```python
from build123d import *

# Parameters (mm, degrees)
F0_W      = 5
F0_H      = 17
F0_H_2    = 8
F0_W_2    = 21
F0_W_3    = 100
F1_DEPTH  = 25
F3_DEPTH  = 8
F4_R      = 2.5
F5_R      = 2.49999
F6_R      = 2.6
F7_DEPTH  = 25
F8_R      = 5
F9_R      = 4.5
F9_R_2    = 2.6
F10_DEPTH = 6
F2_W      = 10
F2_H      = 25
F11_DEPTH = 25
F12_R     = 2


# Not quite as in the source:
# - a fillet or chamfer is up to 0.001 mm smaller than in the source, because OpenCascade refuses the exact size


with BuildPart() as f1:
    # F0 (on Front) → F1 (new body)
    with BuildSketch(Plane.XZ):
        with Locations((-16.2189533483, 16.5)):
            Rectangle(F0_W, F0_H)
        with Locations((-16.2189533483, 4)):
            Rectangle(F0_W, F0_H_2)
        with Locations((-3.2189533483, 4)):
            Rectangle(F0_W_2, F0_H_2)
        with Locations((9.7810466517, 4)):
            Rectangle(F0_W, F0_H_2)
        with Locations((9.7810466517, 16.5)):
            Rectangle(F0_W, F0_H)
        with Locations((62.2810466517, 4)):
            Rectangle(F0_W_3, F0_H_2)
    extrude(amount=F1_DEPTH)

    # F2 (on face) → F3 (join)
    with BuildSketch(Plane.XY.offset(8)):
        Polygon((87.2810466517, -125), (112.2810466517, -125), (112.2810466517, -25), (104.7810466517, -25), (104.7810466517, -115), (94.7810466517, -115), (94.7810466517, -25), (87.2810466517, -25), align=None)
        Polygon((104.7810466517, 0), (112.2810466517, 0), (112.2810466517, 30), (87.2810466517, 30), (87.2810466517, 0), (94.7810466517, 0), (94.7810466517, 20), (104.7810466517, 20), align=None)
    extrude(amount=-F3_DEPTH)

    # F4
    f4_edges = [f1.edges().sort_by_distance(p)[0] for p in [
        (112.281047, -47.5, 0),
        (112.281047, -47.5, 8),
    ]]
    fillet(f4_edges, radius=F4_R)

    # F5 (radius 2.5 in the source; OpenCascade refuses exactly that, so slightly less here)
    f5_edges = [f1.edges().sort_by_distance(p)[0] for p in [
        (12.281047, -12.5, 25),
        (7.281047, -12.5, 25),
        (-18.718953, -12.5, 25),
        (-13.718953, -12.5, 25),
    ]]
    fillet(f5_edges, radius=F5_R)

    # F6 (on face) → F7 (cut)
    with BuildSketch(Plane.XY.offset(8)):
        with Locations((-3.2189533483, -12.5)):
            Circle(F6_R)
    extrude(amount=-F7_DEPTH, mode=Mode.SUBTRACT)

    # F8
    f8_edges = [f1.edges().sort_by_distance(p)[0] for p in [
        (87.281047, 30, 4),
        (87.281047, -125, 4),
    ]]
    fillet(f8_edges, radius=F8_R)

    # F9 (on face) → F10 (cut)
    with BuildSketch(Plane(origin=(0, 0, 0), x_dir=(1, 0, 0), z_dir=(0, 0, -1))):
        with Locations((-3.2189533483, 12.5)):
            Circle(F9_R)
        with Locations((-3.2189533483, 12.5)):
            Circle(F9_R_2, mode=Mode.SUBTRACT)
    extrude(amount=-F10_DEPTH, mode=Mode.SUBTRACT)

    # F2 (on face) → F11 (cut)
    with BuildSketch(Plane.XY.offset(8)):
        with Locations((99.7810466517, -12.5)):
            Rectangle(F2_W, F2_H)
    extrude(amount=-F11_DEPTH, mode=Mode.SUBTRACT)

    # F12
    f12_edges = [f1.edges().sort_by_distance(p)[0] for p in [
        (94.781047, -47.5, 8),
        (99.781047, 20, 8),
        (104.781047, -47.5, 8),
        (99.781047, -115, 8),
        (99.781047, 20, 0),
        (94.781047, -47.5, 0),
        (104.781047, -47.5, 0),
        (99.781047, -115, 0),
    ]]
    fillet(f12_edges, radius=F12_R)


solid = f1.part
```
Model file for the job. Use its own axes, mm. A direction names the side the tool comes from. Coordinates: 2 decimals unless noted, no trailing zeros. Write each loop counter-clockwise with the first axis right and the second up, starting at its lowest first coordinate (ties: lowest second). Pieces come first, ordered by that corner, then holes. Notation, with made-up numbers: (37.5, -20) - (51.5, -20) arc R10 cw to (51.5, -2) - close; hole circle Ø5 at (28.25, -26.75). An arc over 180 degrees is marked (long way). One line per item, written item: value. Start each with the question number.
1. Slice it at D-D (x = 77). Write the cut outline in (y, z), plus the area to 3 significant figures.
2. Tool access for faces 4 (the flat face through (-3.3, -9.6, 6)), 5 (the flat face through (12.281, -12, 15)), 6 (the flat face through (7.281, -12, 15)), 7 (the flat face through (87.281, 13, 4)), 8 (the flat face through (34, -25, 7)): list every direction of +Z, -Z, +X, -X, +Y, -Y with a clear straight run to the whole face (end or side of a thin tool).
3. Slice it at B-B (z = 10.5). Write the cut outline in (x, y).
4. Probe line 1 (X direction, y = -12.5, z = 3.9); line 2 (X direction, y = -21, z = 13); line 3 (X direction, y = -12.5, z = 6.7). List the from-to ranges inside material, lowest first. Write a range as from..to.
5. Mould opens along X. For faces 1 (the flat face through (100, 20, 4)), 2 (the cylindrical face through (88.71, -123.5, 3.94)), 3 (the flat face through (102, -125, 4)) say: released by +X, released by -X, zero draft, split by the parting line, or undercut.
6. Flat gauge pins, fed straight in: pin 1 (4.5 mm diameter, centred on y = -77, z = 4, fed in from -X); pin 2 (5.5 mm diameter, centred on x = -3.22, y = -12.5, fed in from -Z); pin 3 (7.5 mm diameter, centred on y = -18.5, z = 18.5, fed in from +X); pin 4 (23 mm diameter, centred on x = -6, y = -8.5, fed in from +Z). Where does each tip first touch, or does it go through?
7. Slice it at C-C (y = -12.5). Count the separate pieces of the cut face and the enclosed holes in it, plus the area to 3 significant figures.
8. Slice it at A-A (y = -74). Write the cut outline in (x, z), plus the area to 3 significant figures.
Answers below:
1. outline: (-25, 0) - (0, 0) - (0, 8) - (-25, 8) - close
1. area: 200 mm^2
2. face 4: -Z
2. face 5: +Z, +X, +Y, -Y
2. face 6: +Z, +Y, -Y
2. face 7: +Z, -Z, -X, +Y
2. face 8: +Z, -Z, -X, -Y
3. outline: (-18.72, -25) - (-13.72, -25) - (-13.72, 0) - (-18.72, 0) - close; (7.28, -25) - (12.28, -25) - (12.28, 0) - (7.28, 0) - close
4. line 1: x = -18.72..-7.72, 1.28..94.78, 104.78..112.28
4. line 2: x = -18.72..-13.72, 7.28..12.28
4. line 3: x = -18.72..-5.82, -0.62..94.65, 104.91..111.97
5. face 1: undercut
5. face 2: released by -X
5. face 3: zero draft
6. pin 1: stops at x = 87.28
6. pin 2: stops at z = 6
6. pin 3: stops at x = 12.28
6. pin 4: stops at z = 25
7. separate pieces: 3
7. enclosed holes: 0
7. area: 1,060 mm^2
8. outline: (87.28, 0) - (92.78, 0) arc R2 ccw to (94.78, 2) - (94.78, 6) arc R2 ccw to (92.78, 8) - (87.28, 8) - close; (104.78, 2) arc R2 ccw to (106.78, 0) - (109.78, 0) arc R2.5 ccw to (112.28, 2.5) - (112.28, 5.5) arc R2.5 ccw to (109.78, 8) - (106.78, 8) arc R2 ccw to (104.78, 6) - close
8. area: 114 mm^2
